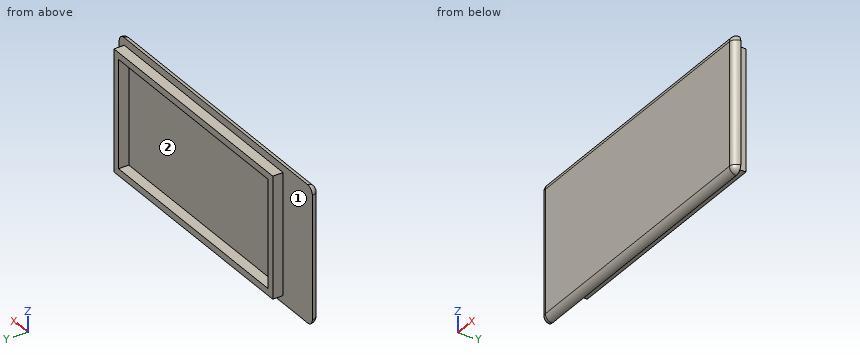
```python
from build123d import *

# Parameters (mm, degrees)
SKETCH1_W           = 42.42562
SKETCH1_H           = 1
BOSS_EXTRUDE1_DEPTH = 19.99996
FILLET1_R           = 1
SKETCH2_W           = 34.8742
SKETCH2_H           = 17.79996
SKETCH2_W_2         = 32.8742
SKETCH2_H_2         = 15.79996
BOSS_EXTRUDE2_DEPTH = 1.5


with BuildPart() as part:
    # Sketch1 → Boss-Extrude1 (new body)
    with BuildSketch(Plane.XY):
        with Locations((21.21281, 0.5)):
            Rectangle(SKETCH1_W, SKETCH1_H)
    extrude(amount=BOSS_EXTRUDE1_DEPTH)

    # Fillet1
    fillet1_edges = [part.edges().sort_by_distance(p)[0] for p in [
        (42.42562, 0.5, 19.99996),
        (0, 0.5, 19.99996),
        (42.42562, 0.5, 0),
        (21.21281, 0, 0),
        (0, 0.5, 0),
        (21.21281, 0, 19.99996),
        (42.42562, 0, 9.99998),
        (0, 0, 9.99998),
    ]]
    fillet(fillet1_edges, radius=FILLET1_R - 0.0001)  # a hair under: the kernel refuses the full size

    # Sketch2 → Boss-Extrude2 (add)
    with BuildSketch(Plane(origin=(0, 1, 0), x_dir=(1, 0, 0), z_dir=(0, 1, 0))):
        with Locations((23.88852, -9.99998)):
            Rectangle(SKETCH2_W, SKETCH2_H)
        with Locations((23.88852, -9.99998)):
            Rectangle(SKETCH2_W_2, SKETCH2_H_2, mode=Mode.SUBTRACT)
    extrude(amount=BOSS_EXTRUDE2_DEPTH)


solid = part.part
```
Verification items for the finished model (mm, model axes). Face numbers are marked on the shaded views. Give positions to 0.01 mm unless a question says otherwise; leave off trailing zeros. Order: outer loops, then holes, each group sorted by start corner. A loop starts at its lowest first (then second) coordinate and runs counter-clockwise, first axis right, second up. Notation, with made-up numbers: M -33.5,22.5 L -2.5,22.5 A12 ccw -2.5,26.5 Z; hole C 25.5,-35.5 d6. An arc over 180 degrees is marked long. Answer in a Markdown table with one row per item. Add a question column.
Item 1: Scan lines: probe 1 along X at (y, z) = (1.5, 16.25); probe 2 along Z at (x, y) = (32.5, 2.15); probe 3 along Y at (x, z) = (11, 1). Record each from-to range of solid material in increasing order. Write a range as from..to.
Item 2: Gauge pin test, flat ends, axial feed: pin 1 (10 mm diameter, centred on x = 30, z = 10, fed in from +Y); pin 2 (1.2 mm diameter, centred on x = 22.5, y = 1.5, fed in from +Z). Record the tip position at first contact, or that the pin passes through.
Item 3: Section check A-A, the plane y = 1.6. Enter the section's corners in (x, z), and give its area (3 significant figures).
Item 4: Mould release check, pull along X, two halves, no side actions. Record for the marked faces 1 and 2: released by +X, released by -X, zero draft, split by the parting line, or undercut.
Filled sheet:
| question | item | result |
|---|---|---|
| 1 | probe 1 | x = 6.45..7.45, 40.33..41.33 |
| 1 | probe 2 | z = 1.1..2.1, 17.9..18.9 |
| 1 | probe 3 | y = 0..1 |
| 2 | pin 1 | stops at y = 1 |
| 2 | pin 2 | stops at z = 20 |
| 3 | outline | M 6.45,1.1 L 41.33,1.1 L 41.33,18.9 L 6.45,18.9 Z; hole M 7.45,2.1 L 40.33,2.1 L 40.33,17.9 L 7.45,17.9 Z |
| 3 | area | 101 mm^2 |
| 4 | face 1 | zero draft |
| 4 | face 2 | undercut |
